Geometry check sheet. Reference: the model listing, model coordinates, mm. Give positions to 0.01 mm unless a question says otherwise; leave off trailing zeros. Order: outer loops, then holes, each group sorted by start corner. A loop starts at its lowest first (then second) coordinate and runs counter-clockwise, first axis right, second up.
Autodesk Inventor part; units mm, degrees
ref_plane "YZ Plane" through (0, 0, 0) normal (1, 0, 0) x (0, 1, 0)
ref_plane "XZ Plane" through (0, 0, 0) normal (0, 1, 0) x (-1, 0, 0)
ref_plane "XY Plane" through (0, 0, 0) normal (0, 0, 1) x (1, 0, 0)
sketch "Sketch1" plane through (0, 0, 0) normal (0, 0, 1) x (1, 0, 0)
  line L0 (0, 0) -> (42.4, 0)
  line L1 (42.4, 0) -> (42.4, 24)
  line L2 (42.4, 24) -> (0, 24)
  line L3 (0, 24) -> (0, 0)
  circle A0 centre (9.2, 20) radius 2.1
  circle A1 centre (33.2, 20) radius 2.1
  circle A2 centre (33.2, 4) radius 2.1
  circle A3 centre (9.2, 4) radius 2.1
  dimension "d0" = 24
  dimension "d1" = 42.4
  dimension "d2" = 4.2
  dimension "d3" = 9.2
  dimension "d4" = 9.2
  dimension "d5" = 9.2
  dimension "d6" = 9.2
  dimension "d7" = 4
  dimension "d8" = 4
  dimension "d9" = 4
  dimension "d10" = 4
extrude "Extrusion1" add sketch "Sketch1" along normal blind 17
sketch "Sketch2" plane through (0, 0, 0) normal (0, -1, 0) x (1, 0, 0)
  line L0 (42.4, 17) -> (0, 17)
  line L1 (0, 0) -> (0, 17)
  circle A0 centre (21.2, 17) radius 4.5
  dimension "d13" = 9
  dimension "d14" = 21.2
  dimension "d15" = 0
extrude "Extrusion2" cut sketch "Sketch2" against normal through all
sketch "Sketch3" plane through (0, 0, 0) normal (0, 0, -1) x (-1, 0, 0)
  arc A0 (-35.3, 4) -> (-35.3, 4) centre (-33.2, 4) ccw
  arc A1 (-11.3, 4) -> (-11.3, 4) centre (-9.2, 4) ccw
  circle A2 centre (-33.2, 20) radius 2.1
  circle A3 centre (-9.2, 20) radius 2.1
  circle A4 centre (-33.2, 20) radius 4.25
  circle A5 centre (-9.2, 20) radius 4.25
  circle A6 centre (-9.2, 4) radius 4.25
  circle A7 centre (-33.2, 4) radius 4.25
  point P0 (0, 0)
  dimension "d20" = 8.5
extrude "Extrusion3" [suppressed]
sketch "Sketch4" plane through (21.2, 0, 17) normal (0, -1, 0) x (1, 0, 0)
  line L0 (-26.3081, 1.9971) -> (24.247, 1.9971)
  line L1 (24.247, 1.9971) -> (24.247, -18.7305)
  line L2 (24.247, -18.7305) -> (-26.3081, -18.7305)
  line L3 (-26.3081, -18.7305) -> (-26.3081, 1.9971)
  point P0 (-21.2, -17)
extrude "Extrusion4" [suppressed]
fillet "Fillet3" radius 3 2 edges at (42.4, 12, 0) (0, 12, 0)
fillet "Fillet4" radius 1 10 edges at (41.5213, 24, 0.8787) (21.2, 24, 0) (42.4, 24, 10) (0.8787, 24, 0.8787) (0, 24, 10) (41.5213, 0, 0.8787) (21.2, 0, 0) (42.4, 0, 10) (0, 0, 10) (0.8787, 0, 0.8787)
sketch "Sketch7" plane through (42.4, 1, 3) normal (1, 0, 0) x (0, 0, -1)
  line L0 (-14, 22) -> (-14, 0)
  circle A0 centre (-6.5, 11) radius 3
  line L1 (0, 23) -> (-14, 23)
  point P0 (3, -1)
  dimension "d35" = 12
  dimension "d36" = 6
  dimension "d37" = 7.5
extrude "Extrusion6" [suppressed]
properties part number "Z move clamp"
Q1. Release check for a two-part mould opening along X. For faces 1 (the face through (0.301, 0.285, 9.902)), 2 (the face through (21, 0, 9)), 3 (the face through (10.33, 18.23, 8.38)) record: pulls with the +X half, pulls with the -X half, needs draft (parallel to the pull), parting line crosses it, or undercut.
Q2. Cross-section at C-C, the plane y = 4. Record the boundary of the cut face in (x, z).
Q3. Cross-section at D-D, the plane z = 8. Record the boundary of the cut face in (x, y).
Q4. Cross-section at B-B, the plane x = 9.2. Record the boundary of the cut face in (y, z).
Q5. Cross-section at A-A, the plane z = 13.5. Record the boundary of the cut face in (x, y), and give its area (3 significant figures).
Q6. Thickness scan on L1, parallel to Y at x = 9, z = 10; L2, parallel to X at y = 21, z = 3; L3, parallel to X at y = 19.75, z = 9.25. Record the ranges inside material, lowest first.
Answers follow:
1. face 1: pulls with the -X half
1. face 2: needs draft
1. face 3: undercut
2. outline: (0, 3) arc R3 ccw to (3, 0) - (7.1, 0) - (7.1, 17) - (0, 17) - close; (11.3, 0) - (31.1, 0) - (31.1, 17) - (25.7, 17) arc R4.5 cw to (16.7, 17) - (11.3, 17) - close; (35.3, 0) - (39.4, 0) arc R3 ccw to (42.4, 3) - (42.4, 17) - (35.3, 17) - close
3. outline: (0, 1) arc R1 ccw to (1, 0) - (41.4, 0) arc R1 ccw to (42.4, 1) - (42.4, 23) arc R1 ccw to (41.4, 24) - (1, 24) arc R1 ccw to (0, 23) - close; hole circle Ø4.2 at (9.2, 4); hole circle Ø4.2 at (9.2, 20); hole circle Ø4.2 at (33.2, 4); hole circle Ø4.2 at (33.2, 20)
4. outline: (0, 1) arc R1 ccw to (1, 0) - (1.9, 0) - (1.9, 17) - (0, 17) - close; (6.1, 0) - (17.9, 0) - (17.9, 17) - (6.1, 17) - close; (22.1, 0) - (23, 0) arc R1 ccw to (24, 1) - (24, 17) - (22.1, 17) - close
5. outline: (0, 1) arc R1 ccw to (1, 0) - (18.37, 0) - (18.37, 24) - (1, 24) arc R1 ccw to (0, 23) - close; (24.03, 0) - (41.4, 0) arc R1 ccw to (42.4, 1) - (42.4, 23) arc R1 ccw to (41.4, 24) - (24.03, 24) - close; hole circle Ø4.2 at (9.2, 4); hole circle Ø4.2 at (9.2, 20); hole circle Ø4.2 at (33.2, 4); hole circle Ø4.2 at (33.2, 20)
5. area: 826 mm2
6. L1: y = 0 to 1.91, 6.09 to 17.91, 22.09 to 24
6. L2: x = 0 to 7.35, 11.05 to 31.35, 35.05 to 42.4
6. L3: x = 0 to 7.11, 11.29 to 31.11, 35.29 to 42.4
